CAD build for the part. Positions are in the model's coordinates, mm. A direction names the side the tool comes from. Give positions to 0.01 mm unless a question says otherwise; leave off trailing zeros. Loops run counter-clockwise (first coordinate to the right, second up) from the corner with the lowest first, then second, coordinate; pieces in that order, holes last. Notation, with made-up numbers: (12, 65) -> (22, 65) arc R35 cw to (22, 97) -> close; hole circle Ø2 at (-19, 50.25). An arc over 180 degrees is marked (long way). Write each question's results on one line, items separated by ' | '. Start each with the question number.
```python
from build123d import *

# Parameters (mm, degrees)
SKETCH1_W           = 127
SKETCH1_H           = 76.2
BOSS_EXTRUDE1_DEPTH = 76.2
SKETCH2_R           = 22.957981207
CUT_EXTRUDE1_DEPTH  = 50.8
CUT_EXTRUDE1_DRAFT  = -15
SKETCH3_R           = 17.955133558
BOSS_EXTRUDE2_DEPTH = 63.5
BOSS_EXTRUDE2_TAPER = 15


with BuildPart() as part:
    # Sketch1 → Boss-Extrude1 (new body)
    with BuildSketch(Plane.XY):
        with Locations((63.5, 38.1)):
            Rectangle(SKETCH1_W, SKETCH1_H)
    extrude(amount=BOSS_EXTRUDE1_DEPTH)


with BuildPart() as cut_extrude1_tool:
    # Sketch2 → Cut-Extrude1 (with draft: the straight prism first)
    with BuildSketch(Plane.XY.offset(76.2)):
        with Locations((64.753202194, 38.155586657)):
            Circle(SKETCH2_R)
    extrude(amount=-CUT_EXTRUDE1_DEPTH)
    # Cut-Extrude1: the draft: its side faces are tilted about the plane it starts from
    cut_extrude1_sides = [cut_extrude1_tool.faces().sort_by_distance(p)[0] for p in [
        (41.795220987, 38.155586657, 50.8),
    ]]
    draft(cut_extrude1_sides, Plane.XY.offset(76.2), CUT_EXTRUDE1_DRAFT)


with BuildPart() as part_1:
    add(part.part)

    # Cut-Extrude1: cut by cut_extrude1_tool
    add(cut_extrude1_tool.part, mode=Mode.SUBTRACT)

    # Sketch3 → Boss-Extrude2 (add)
    with BuildSketch(Plane(origin=(127, 0, 0), x_dir=(0, 0, -1), z_dir=(1, 0, 0))):
        with Locations((-38.791271087, 37.754364457)):
            Circle(SKETCH3_R)
    extrude(amount=BOSS_EXTRUDE2_DEPTH, taper=BOSS_EXTRUDE2_TAPER)


solid = part_1.part
```
Q1. Saw through at B-B, the plane y = 12.5. List the corners of the cut face in (x, z).
Q2. Drop a flat-ended pin along its axis: pin 1 (5 mm diameter, centred on x = 151, z = 47.5, fed in from +Y). Give the stop position or say it passes through.
Q3. Saw through at A-A, the plane z = 64. List the corners of the cut face in (x, y), then the cut area to 3 significant figures.
Q4. Which spindle directions (+Z, -Z, +X, -X, +Y, -Y) get a long thin tool onto all of the face, cutting with end or side? Do faces 5 (the face through (0, 38, 38)), 6 (the face through (65, 38, 25.4)), 7 (the face through (127, 37.6, 20.6)). Say none if no direction does.
Q5. Wall check: L1, parallel to X at y = 67.5, z = 57; L2, parallel to X at y = 52, z = 60; L3, parallel to Y at x = 57.5, z = 73. Give the ranges that are in metal, low to high.
Q6. Saw through at D-D, the plane x = 136. List the corners of the cut face in (y, z), then the cut area to 3 significant figures.
Q7. Mould opens along Y. For faces 1 (the face through (63, 39, 0)), 2 (the face through (61.56, 23.77, 45.51)), 3 (the face through (63, 76.2, 38)), 4 (the face through (159.194, 28.648, 40.814)) say: pulls with the +Y half, pulls with the -Y half, needs draft (parallel to the pull), parting line crosses it, or undercut.
Answer block:
1) outline: (0, 0) -> (127, 0) -> (127, 76.2) -> (0, 76.2) -> close
2) pin 1: stops at y = 47.65
3) outline: (0, 0) -> (127, 0) -> (127, 76.2) -> (0, 76.2) -> close; hole circle Ø39.38 at (64.75, 38.16) | area: 8,460 mm2
4) face 5: +Z, -Z, -X, +Y, -Y | face 6: +Z | face 7: +X
5) L1: x = 0 to 127 | L2: x = 0 to 52.31, 77.2 to 127 | L3: y = 0 to 17.28, 59.03 to 76.2
6) outline: circle Ø31.09 at (37.75, 38.79) | area: 759 mm2
7) face 1: needs draft | face 2: undercut | face 3: pulls with the +Y half | face 4: parting line crosses it
